Autodesk Inventor part; units mm, degrees
ref_plane "YZ Plane" through (0, 0, 0) normal (1, 0, 0) x (0, 1, 0)
ref_plane "XZ Plane" through (0, 0, 0) normal (0, 1, 0) x (-1, 0, 0)
ref_plane "XY Plane" through (0, 0, 0) normal (0, 0, 1) x (1, 0, 0)
sketch "スケッチ1" plane through (0, 0, 0) normal (0, 1, 0) x (-1, 0, 0)
  line L0 (0, 0) -> (-20, 0)
  line L1 (-20, 0) -> (-20, 20)
  line L2 (-20, 20) -> (0, 20)
  line L3 (0, 20) -> (0, 0)
  dimension "d0" = 20
  dimension "d1" = 20
extrude "押し出し1" add sketch "スケッチ1" along normal blind 35
sketch "スケッチ2" plane through (0, 35, 0) normal (0, 1, 0) x (1, 0, 0)
  line L0 (20, 0) -> (0, 0)
  line L1 (0, 0) -> (0, -20)
  line L2 (0, -20) -> (20, -20)
  line L3 (20, -20) -> (20, 0)
  line L4 (0, -10) -> (20, -10)
  line L5 (10, 0) -> (10, -20)
  circle A0 centre (10, -10) radius 4
  line L6 (12.4988, -13.1235) -> (7.5012, -6.8765)
  dimension "d4" = 8
revolve "回転1" add sketch "スケッチ2" angle 360 about axis through (12.4988, 35, 13.1235) along (-0.6246951, 0, -0.7808688) picked at (12.2437, -8.5902) picked at (8.5873, -7.7581) picked at (11.8763, -11.8713) contours A0 L4 L5 | L5 L6 A0 | A0 L6 L4
sketch "スケッチ3" plane through (0, 0, 0) normal (0, -1, 0) x (1, 0, 0)
  line L0 (0, 0) -> (20, 0)
  line L1 (20, 0) -> (20, 20)
  line L2 (20, 20) -> (0, 20)
  line L3 (0, 20) -> (0, 0)
  line L4 (20, 20) -> (0, 0)
  line L5 (0, 20) -> (20, 0)
  point P0 (10, 10)
properties part number "知能ロボコンボールキャスタ"
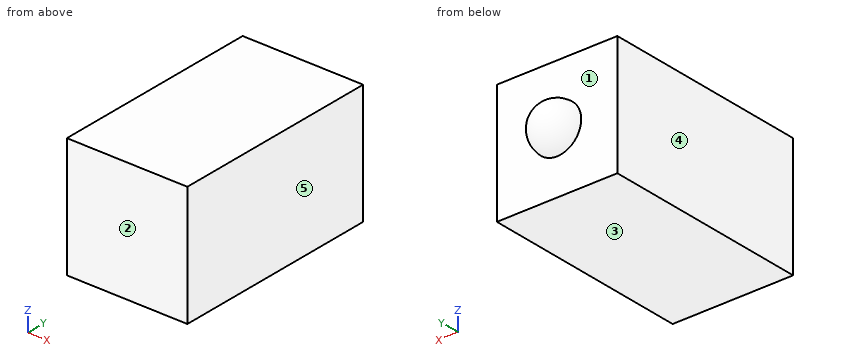
Build history of the part. All positions in model axes, mm. Face numbers are marked on the shaded views. A direction names the side the tool comes from. Round coordinates to 2 decimals unless told otherwise and drop trailing zeros. Write each loop counter-clockwise with the first axis right and the second up, starting at its lowest first coordinate (ties: lowest second). Pieces come first, ordered by that corner, then holes. Notation, with made-up numbers: (74, 24) - (109, 24) arc R17 ccw to (109, 35) - close; hole circle Ø7 at (72.25, 53). An arc over 180 degrees is marked (long way). Use CSV: the item, a comma, the result in double quotes.
(1) 3-axis set-ups, long thin cutter, end or side, ignore diameter. For the marked faces 1 and 2: which of +Z, -Z, +X, -X, +Y, -Y reach the whole face in a straight line?
Response:
face 1,"+Y"
face 2,"+Z, -Z, +X, -X, -Y"
(2) Pin check, flat tip, straight feed: P1, Ø6, axis at x = 6.5, z = 7, coming from the +Y side. Stop position of the tip, or through.
Response:
P1,"y = 38.66"
(3) Band-saw the part on B-B (z = 8). Write the cut outline in (x, y), plus the area to 3 significant figures.
Response:
outline,"(0, 0) - (20, 0) - (20, 35) - (13.46, 35) arc R3.46 ccw to (6.54, 35) - (0, 35) - close"
area,"719 mm²"
(4) Band-saw the part on C-C (z = 2.5). Write the cut outline in (x, y), plus the area to 3 significant figures.
Response:
outline,"(0, 0) - (20, 0) - (20, 35) - (0, 35) - close"
area,"700 mm²"
(5) Band-saw the part on A-A (x = 10.25). Write the cut outline in (y, z), plus the area to 3 significant figures.
Response:
outline,"(0, 0) - (35, 0) - (35, 6.01) arc R3.99 ccw to (35, 13.99) - (35, 20) - (0, 20) - close"
area,"725 mm²"
(6) Wall check: line 1 (Y direction, x = 17.25, z = 18.5); line 2 (Y direction, x = 9, z = 12.5); line 3 (Z direction, x = 10.25, y = 37). Give the ranges that are in metal, low to high.
Response:
line 1,"0 to 35"
line 2,"0 to 37.96"
line 3,"6.54 to 13.46"
(7) Mould opens along X. For the marked faces 3, 4 and 5 say: pulls with the +X half, pulls with the -X half, needs draft (parallel to the pull), parting line crosses it, or undercut.
Response:
face 3,"needs draft"
face 4,"pulls with the -X half"
face 5,"pulls with the +X half"
(8) Band-saw the part on D-D (x = 16.75). Write the cut outline in (y, z).
Response:
outline,"(0, 0) - (35, 0) - (35, 20) - (0, 20) - close"
